Could you check a few things on this model? Use its own coordinates, in mm. Face numbers are marked on the shaded views. A direction names the side the tool comes from. Give positions to 0.01 mm unless a question says otherwise; leave off trailing zeros. Order: outer loops, then holes, each group sorted by start corner. A loop starts at its lowest first (then second) coordinate and runs counter-clockwise, first axis right, second up. Notation, with made-up numbers: (52, -17) - (83, -17) arc R19 ccw to (83, 7) - close; hole circle Ø6 at (36, 57.25). An arc over 180 degrees is marked (long way). Put each result on its own line as item: value.
Autodesk Inventor part; units mm, degrees
ref_plane "YZ Plane" through (0, 0, 0) normal (1, 0, 0) x (0, 1, 0)
ref_plane "XZ Plane" through (0, 0, 0) normal (0, 1, 0) x (-1, 0, 0)
ref_plane "XY Plane" through (0, 0, 0) normal (0, 0, 1) x (1, 0, 0)
sketch "Sketch1" plane through (0, 0, 0) normal (0, 0, 1) x (1, 0, 0)
  circle A0 centre (0, 0) radius 4
  line L0 (2.8868, 5) -> (5.7735, 0)
  line L1 (5.7735, 0) -> (2.8868, -5)
  line L2 (2.8868, -5) -> (-2.8868, -5)
  line L3 (-2.8868, -5) -> (-5.7735, 0)
  line L4 (-5.7735, 0) -> (-2.8868, 5)
  line L5 (-2.8868, 5) -> (2.8868, 5)
  circle A1 centre (0.75, 0) radius 2.65
  dimension "d0" = 8
  dimension "d2" = 10
  dimension "d3" = 5.3
  dimension "d4" = 0.75
extrude "Extrusion1" add sketch "Sketch1" along normal blind 6.35 contours A0 | L0 L1 L2 L3 L4 L5
sketch "Sketch2" plane through (0, 0, 6.35) normal (0, 0, 1) x (1, 0, 0)
  circle A0 centre (0.75, 0) radius 2.65
  circle A1 centre (0, 0) radius 4
  line L0 (4.0415, 7) -> (8.0829, 0)
  line L1 (8.0829, 0) -> (4.0415, -7)
  line L2 (4.0415, -7) -> (-4.0415, -7)
  line L3 (-4.0415, -7) -> (-8.0829, 0)
  line L4 (-8.0829, 0) -> (-4.0415, 7)
  line L5 (-4.0415, 7) -> (4.0415, 7)
  circle A2 centre (0.75, 0) radius 2.65
  dimension "d7" = 8
  dimension "d8" = 14
  dimension "d9" = 5.3
extrude "Extrusion2" add sketch "Sketch2" along normal blind 4.7625 contours A1
properties part number "Eccentric_Spacer"
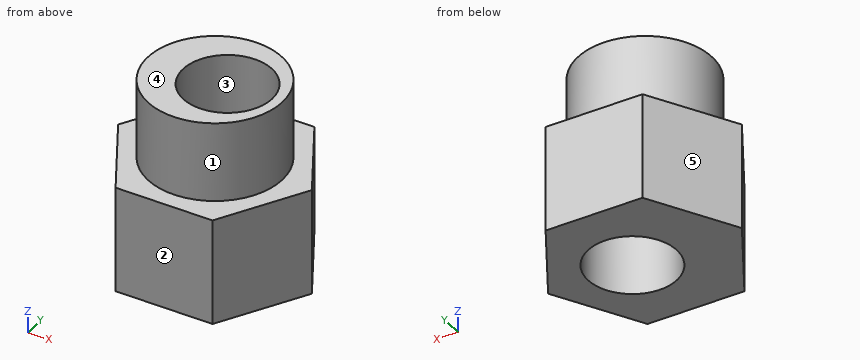
1) Suppose I cut it at D-D, the plane y = -3.5. List the corners of the cut face in (x, z) for me.
Filled in:
outline: (-3.75, 0) - (3.75, 0) - (3.75, 6.35) - (1.94, 6.35) - (1.94, 11.11) - (-1.94, 11.11) - (-1.94, 6.35) - (-3.75, 6.35) - close
2) Suppose I cut it at C-C, the plane y = 1.75. List the corners of the cut face in (x, z) for me.
Filled in:
outline: (-4.76, 0) - (-1.24, 0) - (-1.24, 11.11) - (-3.6, 11.11) - (-3.6, 6.35) - (-4.76, 6.35) - close; (2.74, 0) - (4.76, 0) - (4.76, 6.35) - (3.6, 6.35) - (3.6, 11.11) - (2.74, 11.11) - close
3) Suppose I cut it at B-B, the plane z = 4.5. List the corners of the cut face in (x, y) for me.
Filled in:
outline: (-5.77, 0) - (-2.89, -5) - (2.89, -5) - (5.77, 0) - (2.89, 5) - (-2.89, 5) - close; hole circle Ø5.3 at (0.75, 0)
4) If I drill on line 1 (Y direction, x = 0.75, z = 5); line 2 (Y direction, x = 0.75, z = 7.5); line 3 (Y direction, x = -3, z = 6.5), over which ranges is the centre line in solid material (lowest first)? Write a range as [from, to].
Filled in:
line 1: y = [-5, -2.65], [2.65, 5]
line 2: y = [-3.93, -2.65], [2.65, 3.93]
line 3: y = [-2.65, 2.65]
5) I'm going to push a flat-ended pin straight in: pin 1 (5 mm diameter, centred on x = -0.5, y = 1, fed in from +Z). Where does the tip first touch, or does it pass through?
Filled in:
pin 1: stops at z = 11.11
6) Suppose I cut it at A-A, the plane x = -1.5. List the corners of the cut face in (y, z) for me, and give its area (3 significant figures).
Filled in:
outline: (-5, 0) - (-1.4, 0) - (-1.4, 11.11) - (-3.71, 11.11) - (-3.71, 6.35) - (-5, 6.35) - close; (1.4, 0) - (5, 0) - (5, 6.35) - (3.71, 6.35) - (3.71, 11.11) - (1.4, 11.11) - close
area: 67.7 mm^2
7) Which directions (+Z, -Z, +X, -X, +Y, -Y) give clear straight access to the entire face, cutting with the end or side of a thin tool? Please do the marked faces 1 and 2.
Filled in:
face 1: +Z
face 2: +Z, -Z, +X, -X, -Y
8) We'd pull the mould along Y, two halves only. Please class the marked faces 3, 4 and 5: pulls with the +Y half, pulls with the -Y half, needs draft (parallel to the pull), parting line crosses it, or undercut.
Filled in:
face 3: undercut
face 4: needs draft
face 5: pulls with the +Y half
